Check sheet for the modelled part. Datum: model origin and axes. Units: mm. A direction names the side the tool comes from. Give positions to 0.01 mm unless a question says otherwise; leave off trailing zeros. Order: outer loops, then holes, each group sorted by start corner. A loop starts at its lowest first (then second) coordinate and runs counter-clockwise, first axis right, second up.
```python
from build123d import *

# Parameters (mm, degrees)
SKETCH_1_R      = 31
SKETCH_1_R_2    = 1.5
SKETCH_1_R_3    = 2.75
EXTRUDE_1_DEPTH = 5
SKETCH_1_4_R    = 35
SKETCH_1_4_R_2  = 31
EXTRUDE_3_DEPTH = 20
FILLET_1_R      = 5
FILLET_2_R      = 2
CHAMFER_1_SIZE  = 1
FILLET_3_R      = 3


with BuildPart() as part:
    # Sketch 1 → Extrude 1 (new body)
    with BuildSketch(Plane(origin=(0, 0, 0), x_dir=(1, 0, 0), z_dir=(0, 1, 0))):
        with Locations(Location((0, 0, 0), (0, 0, 270))):
            Circle(SKETCH_1_R)
        with Locations(Location((0, -10, 0), (0, 0, 270))):
            Circle(SKETCH_1_R_2, mode=Mode.SUBTRACT)
        with Locations(Location((10, 0, 0), (0, 0, 270))):
            Circle(SKETCH_1_R_2, mode=Mode.SUBTRACT)
        with Locations(Location((0, 10, 0), (0, 0, 270))):
            Circle(SKETCH_1_R_2, mode=Mode.SUBTRACT)
        with Locations(Location((-10, 0, 0), (0, 0, 270))):
            Circle(SKETCH_1_R_2, mode=Mode.SUBTRACT)
        with Locations(Location((0, 0, 0), (0, 0, 270))):
            Circle(SKETCH_1_R_3, mode=Mode.SUBTRACT)
        with BuildLine():
            ThreePointArc((5, -19.364916731), (14.142135624, -14.142135624), (19.364916731, -5))
            Line((19.364916731, -5), (5, -5))
            Line((5, -5), (5, -19.364916731))
        make_face(mode=Mode.SUBTRACT)
        with BuildLine():
            ThreePointArc((-19.364916731, -5), (-14.142135624, -14.142135624), (-5, -19.364916731))
            Line((-5, -19.364916731), (-5, -5))
            Line((-5, -5), (-19.364916731, -5))
        make_face(mode=Mode.SUBTRACT)
        with BuildLine():
            ThreePointArc((19.364916731, 5), (14.142135624, 14.142135624), (5, 19.364916731))
            Line((5, 19.364916731), (5, 5))
            Line((5, 5), (19.364916731, 5))
        make_face(mode=Mode.SUBTRACT)
        with BuildLine():
            ThreePointArc((-5, 19.364916731), (-14.142135624, 14.142135624), (-19.364916731, 5))
            Line((-19.364916731, 5), (-5, 5))
            Line((-5, 5), (-5, 19.364916731))
        make_face(mode=Mode.SUBTRACT)
    extrude(amount=EXTRUDE_1_DEPTH)

    # Sketch 1_4 → Extrude 3 (add)
    with BuildSketch(Plane(origin=(0, 0, 0), x_dir=(1, 0, 0), z_dir=(0, 1, 0))):
        with Locations(Location((0, 0, 0), (0, 0, 270))):
            Circle(SKETCH_1_4_R)
        with Locations(Location((0, 0, 0), (0, 0, 270))):
            Circle(SKETCH_1_4_R_2, mode=Mode.SUBTRACT)
    extrude(amount=EXTRUDE_3_DEPTH)

    # Fillet 1
    fillet_1_edges = [part.edges().sort_by_distance(p)[0] for p in [
        (-5, 2.5, -5),
        (5, 2.5, -5),
        (-5, 2.5, 5),
        (5, 2.5, 5),
    ]]
    fillet(fillet_1_edges, radius=FILLET_1_R)

    # Fillet 2
    fillet_2_edges = [part.edges().sort_by_distance(p)[0] for p in [
        (-19.364916731, 2.5, -5),
        (-5, 2.5, -19.364916731),
        (5, 2.5, -19.364916731),
        (19.364916731, 2.5, -5),
        (-5, 2.5, 19.364916731),
        (-19.364916731, 2.5, 5),
        (19.364916731, 2.5, 5),
        (5, 2.5, 19.364916731),
    ]]
    fillet(fillet_2_edges, radius=FILLET_2_R)

    # Chamfer 1
    chamfer_1_edges = [part.edges().sort_by_distance(p)[0] for p in [
        (0, 0, -35),
    ]]
    chamfer(chamfer_1_edges, length=CHAMFER_1_SIZE)

    # Fillet 3
    fillet_3_edges = [part.edges().sort_by_distance(p)[0] for p in [
        (0, 5, -31),
    ]]
    fillet(fillet_3_edges, radius=FILLET_3_R)


solid = part.part
```
(1) Sectioned sample at B-B (z = 0). Enter the section's corners in (x, y).
(2) Release check for a two-part mould opening along X. For faces 3 (the face through (-23.2, 20, -20.9)), 4 (the face through (0.07, 2.46, 8.5)), 5 (the face through (0, 5, 6)) record: released by +X, released by -X, zero draft, split by the parting line, or undercut.
(3) Thickness scan on L1, parallel to X at y = 2.65, z = 0; L2, parallel to X at y = 3.1, z = 10; L3, parallel to Y at x = -4, z = -18.5. Record the ranges inside material, lowest first.
(4) Sectioned sample at A-A (y = 4). Count the separate pieces of the cut face and the enclosed holes in it, plus the area to 3 significant figures.
(5) Tool access check on faces 1 (the face through (0, 0, 7)), 2 (the face through (-5.918, 2.535, 18.265)). Record the directions out of +Z, -Z, +X, -X, +Y, -Y that give a thin tool (end or side, any length) a straight path to the whole face; none if there is none.
(6) Sectioned sample at C-C (x = 0). Enter the section's corners in (y, z), plus the area to 3 significant figures.
(7) Sectioned sample at D-D (y = 14.75). Enter the section's corners in (x, z), plus the area to 3 significant figures.
(8) Go/stop test with flat-tipped pins: P1, Ø1.5, axis at x = -26.5, z = -23.5, coming from the -Y side; P2, Ø1.5, axis at x = 14, y = 3, coming from the +Z side (3 decimals); P3, Ø1, axis at x = 19.5, y = 4.5, coming from the +Z side; P4, Ø2.5, axis at x = 0, z = 10, coming from the +Y side. Record where each tip stops, or that it passes through.
Values follow:
1. outline: (-35, 1) - (-34, 0) - (-11.5, 0) - (-11.5, 5) - (-28, 5) arc R3 cw to (-31, 8) - (-31, 20) - (-35, 20) - close; (-8.5, 0) - (-2.75, 0) - (-2.75, 5) - (-8.5, 5) - close; (2.75, 0) - (8.5, 0) - (8.5, 5) - (2.75, 5) - close; (11.5, 0) - (34, 0) - (35, 1) - (35, 20) - (31, 20) - (31, 8) arc R3 cw to (28, 5) - (11.5, 5) - close
2. face 3: zero draft
2. face 4: undercut
2. face 5: undercut
3. L1: x = -35 to -11.5, -8.5 to -2.75, 2.75 to 8.5, 11.5 to 35
3. L2: x = -33.54 to -17.32, -5 to -1.5, 1.5 to 5, 17.32 to 33.54
3. L3: y = 0 to 5
4. separate pieces: 1
4. enclosed holes: 9
4. area: 3,270 mm2
5. face 1: +Z, -Z, +X, -X, -Y
5. face 2: +Y, -Y
6. outline: (0, -34) - (1, -35) - (20, -35) - (20, -31) - (8, -31) arc R3 cw to (5, -28) - (5, -11.5) - (0, -11.5) - close; (0, -8.5) - (5, -8.5) - (5, -2.75) - (0, -2.75) - close; (0, 2.75) - (5, 2.75) - (5, 8.5) - (0, 8.5) - close; (0, 11.5) - (5, 11.5) - (5, 28) arc R3 cw to (8, 31) - (20, 31) - (20, 35) - (1, 35) - (0, 34) - close
6. area: 415 mm2
7. outline: circle Ø70 at (0, 0); hole circle Ø62 at (0, 0)
7. area: 829 mm2
8. P1: stops at y = 0.67
8. P2: stops at z = 32.395
8. P3: stops at z = 29.39
8. P4: passes through
